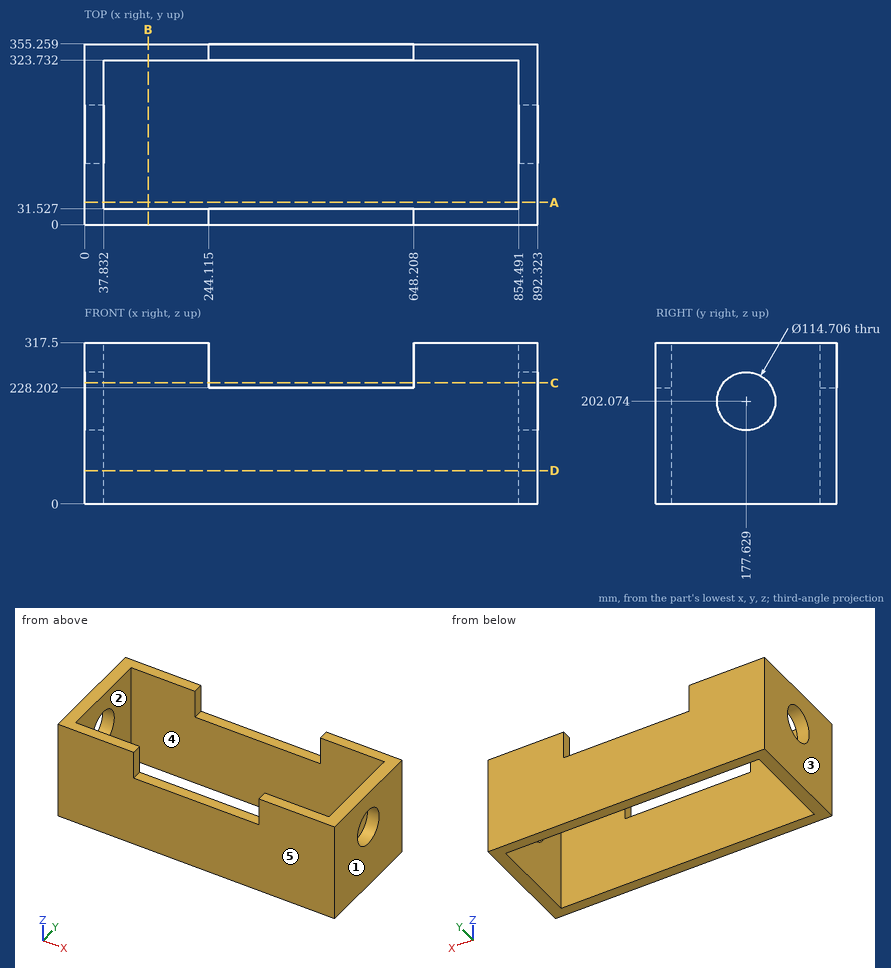
Verification items for this drawing (mm, ordinates from the low corner). A direction names the side the tool comes from. Coordinates: 2 decimals unless noted, no trailing zeros. Loops run counter-clockwise (first coordinate to the right, second up) from the corner with the lowest first, then second, coordinate; pieces in that order, holes last.
Item 1: Access from +Z, -Z, +X, -X, +Y, -Y to the whole of each face (thin tool, end or side, straight path). Record for the marked faces 4 and 5.
Item 2: Sectioned sample at A-A, the plane y = 43.5. Record the boundary of the cut face in (x, z).
Item 3: Thickness scan on line 1 (X direction, y = 137.5, z = 35); line 2 (Y direction, x = 506.5, z = 58); line 3 (X direction, y = 326.5, z = 284) (1 decimal). Record the ranges inside material, lowest first.
Item 4: Sectioned sample at B-B, the plane x = 125. Record the boundary of the cut face in (y, z).
Item 5: Sectioned sample at C-C, the plane z = 238. Record the boundary of the cut face in (x, y) (1 decimal), then the cut area to 3 significant figures.
Item 6: Sectioned sample at D-D, the plane z = 65.5. Record the boundary of the cut face in (x, y).
Item 7: Release check for a two-part mould opening along X. For the marked faces 1, 2 and 3 record: released by +X, released by -X, zero draft, split by the parting line, or undercut.
Check result:
1. face 4: +Z, -Z
1. face 5: +Z, -Z, +X, -X, -Y
2. outline: (0, 0) - (37.83, 0) - (37.83, 317.5) - (0, 317.5) - close; (854.49, 0) - (892.32, 0) - (892.32, 317.5) - (854.49, 317.5) - close
3. line 1: x = 0 to 37.83, 854.49 to 892.32
3. line 2: y = 0 to 31.53, 323.73 to 355.26
3. line 3: x = 0 to 244.1, 648.2 to 892.3
4. outline: (0, 0) - (31.53, 0) - (31.53, 317.5) - (0, 317.5) - close; (323.73, 0) - (355.26, 0) - (355.26, 317.5) - (323.73, 317.5) - close
5. outline: (0, 0) - (244.1, 0) - (244.1, 31.5) - (37.8, 31.5) - (37.8, 132.9) - (0, 132.9) - close; (0, 222.3) - (37.8, 222.3) - (37.8, 323.7) - (244.1, 323.7) - (244.1, 355.3) - (0, 355.3) - close; (648.2, 0) - (892.3, 0) - (892.3, 132.9) - (854.5, 132.9) - (854.5, 31.5) - (648.2, 31.5) - close; (648.2, 323.7) - (854.5, 323.7) - (854.5, 222.3) - (892.3, 222.3) - (892.3, 355.3) - (648.2, 355.3) - close
5. area: 46,100 mm2
6. outline: (0, 0) - (892.32, 0) - (892.32, 355.26) - (0, 355.26) - close; hole (37.83, 31.53) - (854.49, 31.53) - (854.49, 323.73) - (37.83, 323.73) - close
7. face 1: released by +X
7. face 2: undercut
7. face 3: released by -X
